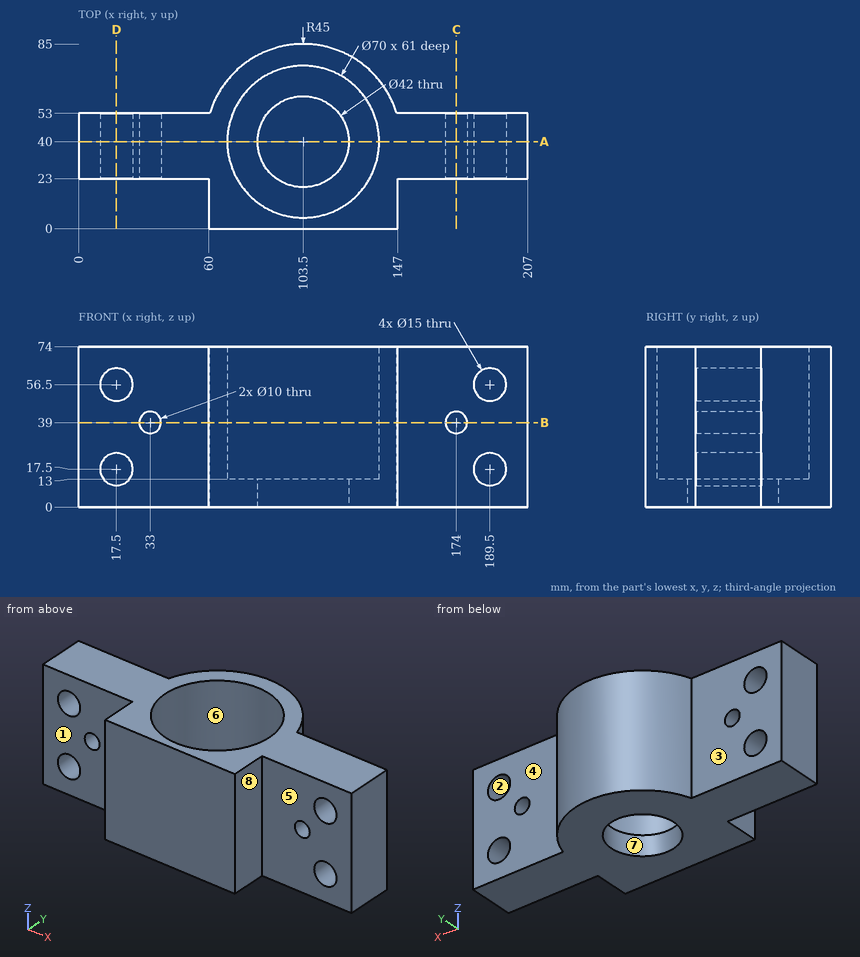
Could you check a few things on this drawing? It's one solid part, dimensions in mm from its lowest x, y, z. A direction names the side the tool comes from. Round coordinates to 2 decimals unless told otherwise and drop trailing zeros. Order: outer loops, then holes, each group sorted by start corner. A loop starts at its lowest first (then second) coordinate and runs counter-clockwise, first axis right, second up.
(1) I'm going to push flat-ended pins straight in: pin 1 (7 mm diameter, centred on y = 12, z = 43.5, fed in from +X); pin 2 (6 mm diameter, centred on x = 130.5, z = 25.5, fed in from +Y); pin 3 (3 mm diameter, centred on x = 53.5, z = 35.5, fed in from +Y). Where does each tip first touch, or does it pass through?
Response values:
pin 1: stops at x = 147
pin 2: stops at y = 78.07
pin 3: stops at y = 53
(2) Imagine slicing it at A-A (y = 40). Write out the boundary of the cut face in (x, z), plus the area to 3 significant figures.
Response values:
outline: (0, 0) - (82.5, 0) - (82.5, 13) - (68.5, 13) - (68.5, 74) - (0, 74) - close; (124.5, 0) - (207, 0) - (207, 74) - (138.5, 74) - (138.5, 13) - (124.5, 13) - close; hole circle Ø15 at (17.5, 17.5); hole circle Ø15 at (17.5, 56.5); hole circle Ø10 at (33, 39); hole circle Ø10 at (174, 39); hole circle Ø15 at (189.5, 17.5); hole circle Ø15 at (189.5, 56.5)
area: 9,640 mm2
(3) Imagine slicing it at C-C (x = 174). Write out the boundary of the cut face in (y, z).
Response values:
outline: (23, 0) - (53, 0) - (53, 34) - (23, 34) - close; (23, 44) - (53, 44) - (53, 74) - (23, 74) - close
(4) Imagine slicing it at B-B (z = 39). Write out the boundary of the cut face in (x, y).
Response values:
outline: (0, 23) - (28, 23) - (28, 53) - (0, 53) - close; (38, 23) - (60, 23) - (60, 0) - (147, 0) - (147, 23) - (169, 23) - (169, 53) - (146.58, 53) arc R45 ccw to (60.42, 53) - (38, 53) - close; (179, 23) - (207, 23) - (207, 53) - (179, 53) - close; hole circle Ø70 at (103.5, 40)
(5) Please list where these lines run through material, in increasing order: line 1 along X through (y, z) = (12, 61.5); line 2 along Y through (x, z) = (103.5, 3.5); line 3 along Z through (x, y) = (16, 34.5).
Response values:
line 1: x = 60 to 82.5, 124.5 to 147
line 2: y = 0 to 19, 61 to 85
line 3: z = 0 to 10.15, 24.85 to 49.15, 63.85 to 74
(6) Which directions (+Z, -Z, +X, -X, +Y, -Y) give clear straight access to the entire face, cutting with the end or side of a thin tool? Please do the marked faces 1, 2, 3 and 4.
Response values:
face 1: +Z, -Z, -X, -Y
face 2: +Y, -Y
face 3: +Z, -Z, -X, +Y
face 4: +Z, -Z, +X, +Y
(7) If we mould it in two halves opening along Y, with no side actions, what happens to the marked faces 5, 6, 7 and 8? For each: released by +Y, released by -Y, zero draft, split by the parting line, or undercut.
Response values:
face 5: released by -Y
face 6: undercut
face 7: undercut
face 8: zero draft
(8) Imagine slicing it at D-D (x = 17.5). Write out the boundary of the cut face in (y, z), plus the area to 3 significant figures.
Response values:
outline: (23, 0) - (53, 0) - (53, 10) - (23, 10) - close; (23, 25) - (53, 25) - (53, 49) - (23, 49) - close; (23, 64) - (53, 64) - (53, 74) - (23, 74) - close
area: 1,320 mm2
